For this review, take the finished solid that the model builds, in its own axes (mm). A direction names the side the tool comes from. Coordinates: 2 decimals unless noted, no trailing zeros. Loops run counter-clockwise (first coordinate to the right, second up) from the corner with the lowest first, then second, coordinate; pieces in that order, holes last. Notation, with made-up numbers: (28.25, 63) - (57.25, 63) arc R13 cw to (57.25, 82) - close; hole circle Ø3 at (1.5, -8). An arc over 180 degrees is marked (long way). Answer as a JSON object with one key per item and string values. Group by question number.
Item 1: Tool access review of faces 1 (the flat face through (1, 0, -38)), 2 (the cylindrical face through (-35.294, 43.344, -5.581)), 3 (the cylindrical face through (-26.706, 53.786, -0.751)): name each direction out of +Z, -Z, +X, -X, +Y, -Y from which nothing blocks a thin tool from reaching the whole face with its end or side.
Item 2: We need section D-D (x = -12.7). Give the boundary of the cut face in (y, z) (3 decimals), then the cut area to 3 significant figures.
Item 3: Mouldability with a two-part tool opening along Y and no side actions: class faces 4 (the flat face through (-47.625, 21, -7)), 5 (the flat face through (1, 76.2, -3)), 6 (the cylindrical face through (27.14, 45.195, -5.581)) as released by +Y, released by -Y, zero draft, split by the parting line, or undercut.
Item 4: We need section A-A (y = 69.85). Give the boundary of the cut face in (x, z) (3 decimals).
Item 5: Clearance check with flat-ended pins moving along their axes: pin 1 (5.5 mm diameter, centred on x = 23.81, y = 46.25, fed in from +Z); pin 2 (10.5 mm diameter, centred on x = -38.1, z = -25.4, fed in from +Y) (3 decimals); pin 3 (20.5 mm diameter, centred on x = 23.81, y = 31.75, fed in from -Z) (3 decimals). State where each tip first meets the part, or that it passes through.
Item 6: To check wall thickness, follow line 1 (Y direction, x = 21, z = -42.5) (3 decimals); line 2 (Z direction, x = -42, y = 55) (3 decimals); line 3 (Z direction, x = -8, y = 38) (3 decimals). State the ranges of each line that lie inside material, in increasing order.
Item 7: We need section B-B (x = 0). Give the boundary of the cut face in (y, z) (3 decimals), then the cut area to 3 significant figures.
Item 8: We need section C-C (z = -50.8). Give the boundary of the cut face in (x, y) (3 decimals).
from build123d import *

# Parameters (mm, degrees)
BOSS_EXTRUDE1_DEPTH     = 47.625
FILLET1_R               = 3.175
F_1_4_20_TAPPED_HOLE1_D = 5.1054
SKETCH6_R               = 8.9408
CUT_EXTRUDE1_DEPTH      = 118.817743252
SKETCH7_R               = 22.225
CUT_EXTRUDE2_DEPTH      = 1.524
F_1_4_20_TAPPED_HOLE2_D = 5.1054
M4_CLEARANCE_HOLE1_D    = 4.3
CUT_EXTRUDE3_DEPTH      = 140.693552859
CIRPATTERN1_START       = -9.525
CIRPATTERN1_DEPTH       = 8.001
F_1_4_CLEARANCE_HOLE1_D = 6.5278


# Read off the part's stored shape, not the designer's step: CirPattern1
with BuildPart() as part:
    # Sketch1 → Boss-Extrude1 (new, symmetric)
    with BuildSketch(Plane(origin=(0, 0, 0), x_dir=(0, 0, -1), z_dir=(1, 0, 0))):
        Polygon((0, 76.2), (0, 0), (76.2, 0), (76.2, 9.525), (9.525, 9.525), (9.525, 76.2), align=None)
    extrude(amount=BOSS_EXTRUDE1_DEPTH, both=True)

    # Fillet1
    fillet1_edges = [part.edges().sort_by_distance(p)[0] for p in [
        (0, 76.2, -9.525),
        (0, 9.525, -9.525),
        (0, 9.525, -76.2),
    ]]
    fillet(fillet1_edges, radius=FILLET1_R)

    # 1/4-20 Tapped Hole1 (through all)
    with Locations(Plane.XY):
        with Locations((-38.1, 69.85), (38.1, 69.85)):
            Hole(F_1_4_20_TAPPED_HOLE1_D / 2)

    # Sketch6 → Cut-Extrude1 (cut, through all)
    with BuildSketch(Plane.XY):
        with Locations((-23.8125, 31.75)):
            Circle(SKETCH6_R)
        with Locations((23.8125, 31.75)):
            Circle(SKETCH6_R)
    extrude(amount=-CUT_EXTRUDE1_DEPTH, mode=Mode.SUBTRACT)

    # Sketch7 → Cut-Extrude2 (cut)
    with BuildSketch(Plane.XY):
        with Locations((-23.8125, 31.75)):
            Circle(SKETCH7_R)
        with Locations((23.8125, 31.75)):
            Circle(SKETCH7_R)
    extrude(amount=-CUT_EXTRUDE2_DEPTH, mode=Mode.SUBTRACT)

    # 1/4-20 Tapped Hole2 (through all)
    with Locations(Plane(origin=(0, 0, -9.525), x_dir=(-1, 0, 0), z_dir=(0, 0, -1))):
        with Locations((0, 41.91)):
            Hole(F_1_4_20_TAPPED_HOLE2_D / 2)

    # M4 Clearance Hole1 (through all)
    with Locations(Plane(origin=(-35.918168185, -13.740381004, -9.525), x_dir=(-1, 0, 0), z_dir=(0, 0, -1))):
        with Locations((-59.730668185, 59.990381004), (-59.730668185, 30.990381004), (-12.105668185, 30.990381004), (-12.105668185, 59.990381004)):
            Hole(M4_CLEARANCE_HOLE1_D / 2)

    # Sketch12 → Cut-Extrude3 (cut, through all)
    with BuildSketch(Plane(origin=(-35.918168185, -13.740381004, -9.525), x_dir=(-1, 0, 0), z_dir=(0, 0, -1))):
        with BuildLine():
            ThreePointArc((-66.626530361, 60.278605165), (-71.268529533, 57.028242353), (-74.518892346, 52.386243181))
            ThreePointArc((-74.518892346, 52.386243181), (-73.228892382, 48.841997409), (-69.68464661, 50.131997373))
            ThreePointArc((-69.68464661, 50.131997373), (-67.496821962, 53.256534782), (-64.372284553, 55.444359429))
            ThreePointArc((-64.372284553, 55.444359429), (-63.082284589, 58.988605201), (-66.626530361, 60.278605165))
        make_face()
    cut_extrude3 = extrude(amount=-CUT_EXTRUDE3_DEPTH, mode=Mode.SUBTRACT)

    # CirPattern1 outline → CirPattern1 (cut)
    with BuildSketch(Plane.XY.offset(CIRPATTERN1_START)):
        with BuildLine():
            ThreePointArc((9.024275839, 38.645862177), (10.314275803, 35.101616405), (13.858521575, 36.391616369))
            ThreePointArc((13.858521575, 36.391616369), (16.046346222, 39.516153778), (19.170883631, 41.703978425))
            ThreePointArc((19.170883631, 41.703978425), (20.460883595, 45.248224197), (16.916637823, 46.538224161))
            ThreePointArc((16.916637823, 46.538224161), (12.274638651, 43.287861349), (9.024275839, 38.645862177))
        make_face()
        with BuildLine():
            ThreePointArc((38.600724161, 24.854137823), (37.310724197, 28.398383595), (33.766478425, 27.108383631))
            ThreePointArc((33.766478425, 27.108383631), (31.578653778, 23.983846222), (28.454116369, 21.796021575))
            ThreePointArc((28.454116369, 21.796021575), (27.164116405, 18.251775803), (30.708362177, 16.961775839))
            ThreePointArc((30.708362177, 16.961775839), (35.350361349, 20.212138651), (38.600724161, 24.854137823))
        make_face()
        with BuildLine():
            ThreePointArc((16.916637823, 16.961775839), (20.460883595, 18.251775803), (19.170883631, 21.796021575))
            ThreePointArc((19.170883631, 21.796021575), (16.046346222, 23.983846222), (13.858521575, 27.108383631))
            ThreePointArc((13.858521575, 27.108383631), (10.314275803, 28.398383595), (9.024275839, 24.854137823))
            ThreePointArc((9.024275839, 24.854137823), (12.274638651, 20.212138651), (16.916637823, 16.961775839))
        make_face()
    cirpattern1 = extrude(amount=CIRPATTERN1_DEPTH, mode=Mode.SUBTRACT)

    # Mirror1: Cut-Extrude3, CirPattern1 across plane
    add(cut_extrude3.mirror(Plane(origin=(0, 0, 0), x_dir=(0, 0, 1), z_dir=(1, 0, 0))), mode=Mode.SUBTRACT)
    add(cirpattern1.mirror(Plane(origin=(0, 0, 0), x_dir=(0, 0, 1), z_dir=(1, 0, 0))), mode=Mode.SUBTRACT)

    # 1/4 Clearance Hole1 (through all)
    with Locations(Plane(origin=(0, 9.525, 0), x_dir=(1, 0, 0), z_dir=(0, 1, 0))):
        with Locations((-38.1, 25.4), (38.1, 25.4), (-12.7, 50.8), (12.7, 50.8)):
            Hole(F_1_4_CLEARANCE_HOLE1_D / 2)


solid = part.part
Check sheet entries:
{
 "1": {"face 1": "+Z, -Z, +X, -X, -Y", "face 2": "+Z, -Z", "face 3": "+Z"},
 "2": {"outline": "(0, -76.2) - (6.35, -76.2) arc R3.175 ccw to (9.525, -73.025) - (9.525, -54.064) - (0, -54.064) - close; (0, -47.536) - (9.525, -47.536) - (9.525, -12.7) arc R3.175 cw to (12.7, -9.525) - (19.802, -9.525) - (19.802, -1.524) - (12.503, -1.524) - (12.503, 0) - (0, 0) - close; (28.333, -9.525) - (35.167, -9.525) - (35.167, -1.524) - (28.333, -1.524) - close; (43.698, -9.525) - (73.025, -9.525) arc R3.175 ccw to (76.2, -6.35) - (76.2, 0) - (50.997, 0) - (50.997, -1.524) - (43.698, -1.524) - close", "area": "1,100 mm2"},
 "3": {"face 4": "zero draft", "face 5": "released by +Y", "face 6": "undercut"},
 "4": {"outline": "(-47.625, -9.525) - (-40.653, -9.525) - (-40.653, 0) - (-47.625, 0) - close; (-35.547, -9.525) - (35.547, -9.525) - (35.547, 0) - (-35.547, 0) - close; (40.653, -9.525) - (47.625, -9.525) - (47.625, 0) - (40.653, 0) - close"},
 "5": {"pin 1": "stops at z = -1.52", "pin 2": "stops at y = 9.525", "pin 3": "stops at z = -9.525"},
 "6": {"line 1": "y = 0 to 9.525", "line 2": "z = -9.525 to 0", "line 3": "z = -9.525 to -1.524"},
 "7": {"outline": "(0, -76.2) - (6.35, -76.2) arc R3.175 ccw to (9.525, -73.025) - (9.525, -12.7) arc R3.175 cw to (12.7, -9.525) - (39.357, -9.525) - (39.357, 0) - (0, 0) - close; (44.463, -9.525) - (73.025, -9.525) arc R3.175 ccw to (76.2, -6.35) - (76.2, 0) - (44.463, 0) - close", "area": "1,310 mm2"},
 "8": {"outline": "(-47.625, 0) - (-15.964, 0) - (-15.964, 9.525) - (-47.625, 9.525) - close; (-9.436, 0) - (9.436, 0) - (9.436, 9.525) - (-9.436, 9.525) - close; (15.964, 0) - (47.625, 0) - (47.625, 9.525) - (15.964, 9.525) - close"}
}
